from build123d import *

# Parameters (mm, degrees)
SKETCH1_W               = 8
SKETCH1_H               = 8
BOSS_EXTRUDE1_DEPTH     = 3
CUT_EXTRUDE1_DEPTH      = 12.704699911
CUT_EXTRUDE1_DEPTH_BACK = 12.704699911
CUT_EXTRUDE2_DEPTH      = 11
SKETCH4_R               = 1.75
CUT_EXTRUDE3_DEPTH      = 0.4
SKETCH5_W               = 8
SKETCH5_H               = 1
BOSS_EXTRUDE2_DEPTH     = 2
FILLET1_R               = 4
CUT_EXTRUDE4_DEPTH      = 0.4


with BuildPart() as part:
    # Sketch1 → Boss-Extrude1 (new body)
    with BuildSketch(Plane(origin=(0, 0, 0), x_dir=(1, 0, 0), z_dir=(0, 1, 0))):
        with Locations((4, 4)):
            Rectangle(SKETCH1_W, SKETCH1_H)
    extrude(amount=BOSS_EXTRUDE1_DEPTH)

    # Sketch2 → Cut-Extrude1 (cut, two sides: drawn at the far end of the back side and taken through both)
    with BuildSketch(Plane.XY.offset(-CUT_EXTRUDE1_DEPTH_BACK)):
        Polygon((0, 0), (0.6, 3), (0, 3), align=None)
        Polygon((8, 0), (7.4, 3), (8, 3), align=None)
    extrude(amount=CUT_EXTRUDE1_DEPTH + CUT_EXTRUDE1_DEPTH_BACK, mode=Mode.SUBTRACT)

    # Sketch3 → Cut-Extrude2 (cut)
    with BuildSketch(Plane(origin=(0, 0, 0), x_dir=(0, 0, -1), z_dir=(1, 0, 0))):
        Polygon((0, 0), (0.6, 3), (0, 3), align=None)
        Polygon((8, 3), (7.4, 3), (8, 0), align=None)
    extrude(amount=CUT_EXTRUDE2_DEPTH, mode=Mode.SUBTRACT)

    # Sketch4 → Cut-Extrude3 (cut)
    with BuildSketch(Plane.XZ):
        with Locations(Location((4, -3.75, 0), (0, 0, 270))):
            Circle(SKETCH4_R)
    extrude(amount=-CUT_EXTRUDE3_DEPTH, mode=Mode.SUBTRACT)

    # Sketch5 → Boss-Extrude2 (add)
    with BuildSketch(Plane.XZ):
        with Locations((4, -7.5)):
            Rectangle(SKETCH5_W, SKETCH5_H)
    extrude(amount=BOSS_EXTRUDE2_DEPTH)

    # Fillet1
    # the kernel refuses this fillet: 4 mm, written as the material it takes off along each edge
    with BuildSketch(Plane(origin=(8, -2, -16.660254038), x_dir=(0, 1, 0), z_dir=(0, 0, 1)), Plane(origin=(0, -2, 1.660254038), x_dir=(0, 1, 0), z_dir=(0, 0, -1))) as fillet1_piece_1:
        with BuildLine():
            CenterArc((4, 3.464101615), FILLET1_R, 180, 60)
            Line((0, 3.464101615), (-0.08, 3.464101615))
            Line((-0.08, 3.464101615), (-0.08, 0))
            Line((-0.08, 0), (0, -0.08))
            ThreePointArc((0, -0.08), (1, -0.08), (1.96, -0.069282032))
            Line((1.96, -0.069282032), (2, 0))
        make_face()
    extrude(amount=18.320508076, mode=Mode.SUBTRACT)

    # Sketch6 → Cut-Extrude4 (cut)
    with BuildSketch(Plane(origin=(0, 3, 0), x_dir=(1, 0, 0), z_dir=(0, 1, 0))):
        with BuildLine():
            Line((2.366875023, 6.025988971), (3.978253228, 6.025988971))
            add(Edge.make_bspline(
                [(3.978253228, 6.025988971), (4.016981522, 6.025758539), (4.091770291, 6.025313549), (4.200234262, 6.02407341), (4.300910244, 6.020431423), (4.393955008, 6.01730407), (4.479059098, 6.009990491), (4.556891378, 6.004244483), (4.627206795, 5.996339471), (4.710040188, 5.983546816), (4.806360793, 5.963648743), (4.915152558, 5.926842691), (5.018276483, 5.880857129), (5.114182519, 5.822393524), (5.203189243, 5.754016663), (5.28597738, 5.676271174), (5.358728101, 5.58601543), (5.424238976, 5.487508268), (5.479534837, 5.380666952), (5.517612886, 5.26572697), (5.541913225, 5.144795761), (5.544858568, 5.061898711), (5.546362202, 5.019578715)],
                knots=[0, 0, 0, 0, 1.096610875, 2.117681168, 3.071055591, 3.949137991, 4.753059115, 5.489127199, 6.15892391, 6.75575099, 7.862330316, 8.938514814, 10.001276227, 11.05313779, 12.110449801, 13.174958802, 14.260456508, 15.384725817, 16.521138801, 17.654729897, 18.802709851, 20, 20, 20, 20], degree=3))
            add(Edge.make_bspline(
                [(5.546362202, 5.019578715), (5.544802721, 4.973493311), (5.541727769, 4.882623117), (5.513106772, 4.749371009), (5.467516851, 4.621879661), (5.40315043, 4.502217288), (5.324314646, 4.392405777), (5.231065087, 4.295977947), (5.12477188, 4.213520097), (5.044958184, 4.17248881), (5.004695536, 4.151790253)],
                knots=[0, 0, 0, 0, 1.023065178, 2.01725758, 3.014298905, 4.023406433, 5.026736079, 6.009055718, 6.99565244, 8, 8, 8, 8], degree=3))
            add(Edge.make_bspline(
                [(5.004695536, 4.151790253), (5.0318132, 4.142553707), (5.085431798, 4.12429068), (5.162178571, 4.090754541), (5.234086142, 4.051862796), (5.301118401, 4.008841827), (5.363784101, 3.961377137), (5.420252395, 3.907894911), (5.473763466, 3.851437899), (5.520742036, 3.789172127), (5.563264851, 3.724075672), (5.599360366, 3.65512964), (5.630616076, 3.583992364), (5.656755805, 3.509943884), (5.675388869, 3.432487562), (5.69031884, 3.352599145), (5.697956597, 3.269724954), (5.699451608, 3.213768347), (5.700208356, 3.185444099)],
                knots=[0, 0, 0, 0, 1.072651974, 2.1209089, 3.132484228, 4.131466326, 5.101889999, 6.071643115, 7.041396231, 8.011819904, 8.988565287, 9.95070344, 10.922775742, 11.897213062, 12.887138018, 13.903598663, 14.938838629, 16, 16, 16, 16], degree=3))
            add(Edge.make_bspline(
                [(5.700208356, 3.185444099), (5.698598844, 3.140212221), (5.695387249, 3.049957264), (5.671387404, 2.915316113), (5.630853991, 2.783046233), (5.575963383, 2.654005704), (5.507783193, 2.532330941), (5.427626978, 2.4212421), (5.334105775, 2.324584109), (5.230539132, 2.239414342), (5.113835126, 2.16890592), (4.984093466, 2.114745557), (4.842134035, 2.073828468), (4.742124288, 2.060236169), (4.690592972, 2.053232561)],
                knots=[0, 0, 0, 0, 0.975059807, 1.945618526, 2.93861228, 3.952760547, 4.963632603, 5.940527786, 6.897802811, 7.855787948, 8.824773195, 9.82606706, 10.879852914, 12, 12, 12, 12], degree=3))
            add(Edge.make_bspline(
                [(4.690592972, 2.053232561), (4.670833027, 2.051565703), (4.625472552, 2.047739302), (4.548543711, 2.042982046), (4.453955886, 2.039386091), (4.341791209, 2.035134329), (4.211704387, 2.032064432), (4.063991072, 2.029968108), (3.898399223, 2.027247493), (3.782207382, 2.026423), (3.72104169, 2.025988971)],
                knots=[0, 0, 0, 0, 0.490565993, 1.126131979, 1.906526787, 2.832178623, 3.902933831, 5.125497984, 6.486805064, 8, 8, 8, 8], degree=3))
            Line((3.72104169, 2.025988971), (2.366875023, 2.025988971))
            Line((2.366875023, 2.025988971), (2.366875023, 6.025988971))
        make_face()
        with BuildLine():
            Line((3.136105792, 5.359322304), (3.136105792, 4.436245381))
            Line((3.136105792, 4.436245381), (3.692996818, 4.436245381))
            add(Edge.make_bspline(
                [(3.692996818, 4.436245381), (3.732259986, 4.43615888), (3.807047978, 4.435994114), (3.91334909, 4.43709824), (4.008173732, 4.437613694), (4.091249283, 4.439126475), (4.162558686, 4.441623123), (4.221845003, 4.444116229), (4.269450826, 4.446003799), (4.297170592, 4.448699163), (4.309182715, 4.449867176)],
                knots=[0, 0, 0, 0, 1.528479216, 2.911428072, 4.138414629, 5.21998762, 6.145918986, 6.915989543, 7.530253335, 8, 8, 8, 8], degree=3))
            add(Edge.make_bspline(
                [(4.309182715, 4.449867176), (4.3438238, 4.455079871), (4.41040184, 4.465098351), (4.503567155, 4.494454854), (4.584375726, 4.536913614), (4.653724553, 4.58976356), (4.708773054, 4.654604252), (4.749170144, 4.72919452), (4.772805412, 4.813847791), (4.775653451, 4.873327339), (4.777131433, 4.904194099)],
                knots=[0, 0, 0, 0, 1.162079002, 2.233444551, 3.225172046, 4.179556897, 5.110707885, 6.027301426, 6.976273101, 8, 8, 8, 8], degree=3))
            add(Edge.make_bspline(
                [(4.777131433, 4.904194099), (4.776203651, 4.934000177), (4.774422539, 4.991220438), (4.752297006, 5.072236392), (4.719032932, 5.144995211), (4.670409719, 5.207709385), (4.609395094, 5.260672186), (4.534716376, 5.302043411), (4.446732173, 5.330510733), (4.38335661, 5.340467498), (4.3500481, 5.345700509)],
                knots=[0, 0, 0, 0, 1.044241546, 2.004684189, 2.928111627, 3.838334562, 4.769594837, 5.748424953, 6.81663206, 8, 8, 8, 8], degree=3))
            add(Edge.make_bspline(
                [(4.3500481, 5.345700509), (4.336967148, 5.34687206), (4.306041436, 5.349641817), (4.252292165, 5.35144236), (4.183926257, 5.353976507), (4.100595234, 5.356449705), (4.002296842, 5.357959731), (3.889310645, 5.358468661), (3.761641688, 5.359577608), (3.671629596, 5.359410545), (3.624086561, 5.359322304)],
                knots=[0, 0, 0, 0, 0.433943041, 1.02591908, 1.776648879, 2.694999143, 3.780816848, 5.02540149, 6.428861738, 8, 8, 8, 8], degree=3))
            Line((3.624086561, 5.359322304), (3.136105792, 5.359322304))
        make_face(mode=Mode.SUBTRACT)
        with BuildLine():
            Line((3.136105792, 3.769578715), (3.136105792, 2.692655638))
            Line((3.136105792, 2.692655638), (3.921362202, 2.692655638))
            add(Edge.make_bspline(
                [(3.921362202, 2.692655638), (3.957955896, 2.692474114), (4.027408125, 2.692129595), (4.126486109, 2.694437139), (4.214933064, 2.69519802), (4.293162962, 2.698994102), (4.360764719, 2.701865798), (4.418016495, 2.705445849), (4.464471269, 2.711139165), (4.491885355, 2.715559172), (4.503894254, 2.717495381)],
                knots=[0, 0, 0, 0, 1.504773752, 2.85595359, 4.075347731, 5.141676974, 6.076328919, 6.858106537, 7.499786952, 8, 8, 8, 8], degree=3))
            add(Edge.make_bspline(
                [(4.503894254, 2.717495381), (4.534390702, 2.723929926), (4.593642924, 2.736431746), (4.675765739, 2.772305806), (4.749780788, 2.817800627), (4.813883543, 2.876271003), (4.866572685, 2.946316906), (4.904617992, 3.02809262), (4.927561873, 3.120636015), (4.929805566, 3.185839411), (4.930977587, 3.219899227)],
                knots=[0, 0, 0, 0, 1.031056579, 2.003262591, 2.954260215, 3.900917722, 4.862741126, 5.841340256, 6.872396835, 8, 8, 8, 8], degree=3))
            add(Edge.make_bspline(
                [(4.930977587, 3.219899227), (4.930031736, 3.249108452), (4.928190747, 3.305960799), (4.910169932, 3.38739087), (4.88101832, 3.461844609), (4.840421058, 3.528813936), (4.789699747, 3.589139928), (4.726998003, 3.639624345), (4.654607383, 3.681685756), (4.585597801, 3.709395341), (4.520158829, 3.72717269), (4.457743787, 3.73883498), (4.382520906, 3.748066566), (4.294854864, 3.755875466), (4.194389919, 3.762120128), (4.081396073, 3.767043008), (3.95555801, 3.769103428), (3.867409493, 3.769415255), (3.821201946, 3.769578715)],
                knots=[0, 0, 0, 0, 0.992165387, 1.931134082, 2.820086661, 3.700270762, 4.583075858, 5.486803518, 6.423132184, 7.421722103, 8.005700193, 8.727213115, 9.57900282, 10.582332745, 11.720121093, 13.002085041, 14.428489784, 16, 16, 16, 16], degree=3))
            Line((3.821201946, 3.769578715), (3.136105792, 3.769578715))
        make_face(mode=Mode.SUBTRACT)
    extrude(amount=-CUT_EXTRUDE4_DEPTH, mode=Mode.SUBTRACT)


solid = part.part
Input: part model. Units: mm. Frame: model coordinates. A direction names the side the tool comes from. Coordinates: 2 decimals unless noted, no trailing zeros. Order: outer loops, then holes, each group sorted by start corner. A loop starts at its lowest first (then second) coordinate and runs counter-clockwise, first axis right, second up.
1. Cut plane A-A, the plane y = 0.1. Return loops of the section in (x, z), plus the area to 3 significant figures.
Checked values:
outline: (0.02, -7.98) - (7.98, -7.98) - (7.98, -0.02) - (0.02, -0.02) - close; hole circle Ø3.5 at (4, -3.75)
area: 53.7 mm2
2. Draft query along X for faces 1 (the flat face through (4, 3, -3)), 2 (the flat face through (4, 2.6, -4)), 3 (the cylindrical face through (6.51, -1.48, -7.51)). Return one class per face: +X half, -X half, draft (parallel to the pull), parting line (faces both ways), or undercut.
Checked values:
face 1: draft
face 2: undercut
face 3: +X half
3. Cut plane C-C, the plane z = -7.5. Return loops of the section in (x, y), plus the area to 3 significant figures.
Checked values:
outline: (0, 0) arc R4 ccw to (3.46, -2) - (4.54, -2) arc R4 ccw to (8, 0) - (7.5, 2.5) - (0.5, 2.5) - close
area: 30.7 mm2
4. Access query for faces 4 (the flat face through (7.7, 1.5, -4.1)), 5 (the flat face through (3, 0, -2)), 6 (the flat face through (4, 0.4, -4)). Directions: +Z, -Z, +X, -X, +Y, -Y. A direction counts if a zero-diameter tool reaches every point of the face in a straight line with its end or side. Return the directions, or none.
Checked values:
face 4: +Z, -Z, +X, +Y
face 5: +Z, +X, -X, -Y
face 6: -Y
5. Cut plane D-D, the plane y = 1.5. Return loops of the section in (x, z).
Checked values:
outline: (0.3, -7.7) - (7.7, -7.7) - (7.7, -0.3) - (0.3, -0.3) - close
6. Ray query, line 1 along Y through (x, z) = (5.75, -5.5); line 2 along Z through (x, y) = (5, -0.8); line 3 along Z through (x, y) = (4.5, 0.15). Return the intervals inside material, ascending.
Checked values:
line 1: y = 0 to 3
line 2: z = -8 to -7
line 3: z = -7.97 to -5.43, -2.07 to -0.03
7. Contact query for flat-ended pins moving along their axis: P1, Ø3.5, axis at x = 4.5, z = -3, coming from the -Y side; P2, Ø1.8, axis at x = 4, z = -4, coming from the -Y side; P3, Ø1, axis at y = 1, z = -2.5, coming from the -X side. Output: stop coordinate, or through.
Checked values:
P1: stops at y = 0
P2: stops at y = 0.4
P3: stops at x = 0.1
8. Cut plane B-B, the plane x = 2.5. Return loops of the section in (y, z), plus the area to 3 significant figures.
Checked values:
outline: (-1.88, -8) - (0, -8) - (3, -7.4) - (3, -6.03) - (2.6, -6.03) - (2.6, -2.03) - (3, -2.03) - (3, -0.6) - (0, 0) - (0, -2.85) - (0.4, -2.85) - (0.4, -4.65) - (0, -4.65) - (0, -7) - (-1.88, -7) - close
area: 21.8 mm2
